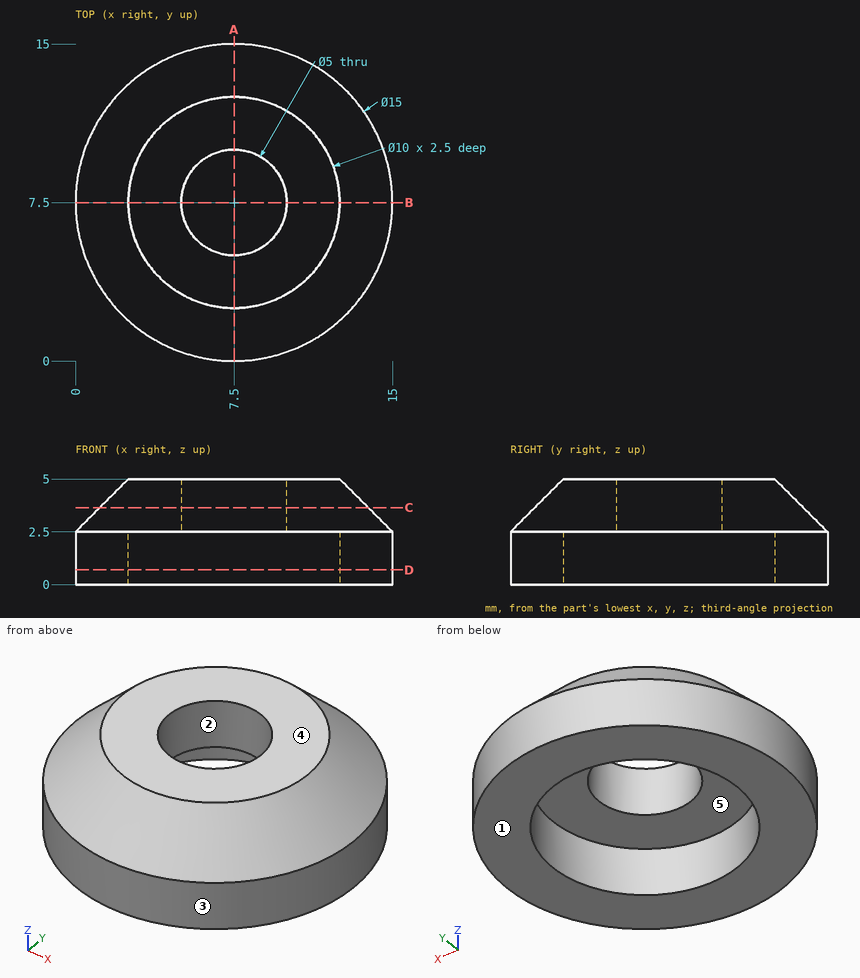
Could you check a few things on this drawing? It's one solid part, dimensions in mm from its lowest x, y, z. A direction names the side the tool comes from. Round coordinates to 2 decimals unless told otherwise and drop trailing zeros. Loops run counter-clockwise (first coordinate to the right, second up) from the corner with the lowest first, then second, coordinate; pieces in that order, holes last. Notation, with made-up numbers: (87, -23) -> (118, -23) arc R17 ccw to (118, 0) -> close; hole circle Ø7 at (62, 79). An arc over 180 degrees is marked (long way). One line per item, written item: value. Start each with the question number.
1. If we section it at A-A, the plane x = 7.5: Write out the boundary of the cut face in (y, z), then the cut area to 4 significant figures.
2. If we section it at C-C, the plane z = 3.65: Write out the boundary of the cut face in (x, y).
3. If I drill on probe 1 along Y at (x, z) = (7.5, 1.7); probe 2 along Z at (x, y) = (3.5, 8.5); probe 3 along X at (y, z) = (10.25, 1.15), over which ranges is the centre line in solid material (lowest first)?
4. For the marked faces 4 and 5, which set-ups out of +Z, -Z, +X, -X, +Y, -Y let a thin tool reach every point of the face, with its end or its side?
5. If we section it at D-D, the plane z = 0.7: Write out the boundary of the cut face in (x, y), then the cut area to 3 significant figures.
6. For pin 1 (5 mm diameter, centred on x = 8.5, y = 7, fed in from -Z); pin 2 (1.5 mm diameter, centred on x = 1.5, y = 5, fed in from +Z), each with a flat end and sliding along its axis, tell me the tip position at first contact or that it passes through.
7. If we mould it in two halves opening along Y, with no side actions, what happens to the marked faces 1, 2 and 3? For each: pulls with the +Y half, pulls with the -Y half, needs draft (parallel to the pull), parting line crosses it, or undercut.
Calculated:
1. outline: (0, 0) -> (2.5, 0) -> (2.5, 2.5) -> (5, 2.5) -> (5, 5) -> (2.5, 5) -> (0, 2.5) -> close; (10, 2.5) -> (12.5, 2.5) -> (12.5, 0) -> (15, 0) -> (15, 2.5) -> (12.5, 5) -> (10, 5) -> close
1. area: 31.25 mm²
2. outline: circle Ø12.7 at (7.5, 7.5); hole circle Ø5 at (7.5, 7.5)
3. probe 1: y = 0 to 2.5, 12.5 to 15
3. probe 2: z = 2.5 to 5
3. probe 3: x = 0.52 to 3.32, 11.68 to 14.48
4. face 4: +Z, +X, -X, +Y, -Y
4. face 5: -Z
5. outline: circle Ø15 at (7.5, 7.5); hole circle Ø10 at (7.5, 7.5)
5. area: 98.2 mm²
6. pin 1: stops at z = 2.5
6. pin 2: stops at z = 4.25
7. face 1: needs draft
7. face 2: undercut
7. face 3: parting line crosses it
